```python
from build123d import *

# Parameters (mm, degrees)
F0_R     = 65
F0_R_2   = 5.5
F0_R_3   = 12
F1_DEPTH = 52
F0_R_4   = 81.25
F0_R_5   = 4
F2_DEPTH = 13
F3_DEPTH = 5.2


with BuildPart() as f1:
    # F0 (on Right) → F1 (new body)
    with BuildSketch(Plane.YZ):
        Circle(F0_R)
        with Locations((-28.145826, -16.25)):
            Circle(F0_R_2, mode=Mode.SUBTRACT)
        with Locations((0, -32.5)):
            Circle(F0_R_2, mode=Mode.SUBTRACT)
        with Locations((28.145826, -16.25)):
            Circle(F0_R_2, mode=Mode.SUBTRACT)
        with Locations((-28.145826, 16.25)):
            Circle(F0_R_2, mode=Mode.SUBTRACT)
        Circle(F0_R_3, mode=Mode.SUBTRACT)
        with Locations((28.145826, 16.25)):
            Circle(F0_R_2, mode=Mode.SUBTRACT)
        with Locations((0, 32.5)):
            Circle(F0_R_2, mode=Mode.SUBTRACT)
    extrude(amount=F1_DEPTH)

    # F0 (on Right) → F2 (join)
    with BuildSketch(Plane.YZ):
        Circle(F0_R_4)
        with Locations((-47.013486, -56.028491)):
            Circle(F0_R_5, mode=Mode.SUBTRACT)
        with Locations((-25.015353, -68.729118)):
            Circle(F0_R_5, mode=Mode.SUBTRACT)
        with Locations((-63.341098, -36.57)):
            Circle(F0_R_5, mode=Mode.SUBTRACT)
        with Locations((-72.028839, -12.700628)):
            Circle(F0_R_5, mode=Mode.SUBTRACT)
        with Locations((0, -73.14)):
            Circle(F0_R_5, mode=Mode.SUBTRACT)
        with Locations((25.015353, -68.729118)):
            Circle(F0_R_5, mode=Mode.SUBTRACT)
        with Locations((47.013486, -56.028491)):
            Circle(F0_R_5, mode=Mode.SUBTRACT)
        with Locations((63.341098, -36.57)):
            Circle(F0_R_5, mode=Mode.SUBTRACT)
        with Locations((72.028839, -12.700628)):
            Circle(F0_R_5, mode=Mode.SUBTRACT)
        with Locations((-72.028839, 12.700628)):
            Circle(F0_R_5, mode=Mode.SUBTRACT)
        with Locations((-63.341098, 36.57)):
            Circle(F0_R_5, mode=Mode.SUBTRACT)
        with Locations((-47.013486, 56.028491)):
            Circle(F0_R_5, mode=Mode.SUBTRACT)
        with Locations((-25.015353, 68.729118)):
            Circle(F0_R_5, mode=Mode.SUBTRACT)
        Circle(F0_R, mode=Mode.SUBTRACT)
        with Locations((72.028839, 12.700628)):
            Circle(F0_R_5, mode=Mode.SUBTRACT)
        with Locations((63.341098, 36.57)):
            Circle(F0_R_5, mode=Mode.SUBTRACT)
        with Locations((0, 73.14)):
            Circle(F0_R_5, mode=Mode.SUBTRACT)
        with Locations((25.015353, 68.729118)):
            Circle(F0_R_5, mode=Mode.SUBTRACT)
        with Locations((47.013486, 56.028491)):
            Circle(F0_R_5, mode=Mode.SUBTRACT)
    extrude(amount=F2_DEPTH)

    # F0 (on Right) → F3 (join)
    with BuildSketch(Plane.YZ):
        Circle(F0_R)
        with Locations((-28.145826, -16.25)):
            Circle(F0_R_2, mode=Mode.SUBTRACT)
        with Locations((0, -32.5)):
            Circle(F0_R_2, mode=Mode.SUBTRACT)
        with Locations((28.145826, -16.25)):
            Circle(F0_R_2, mode=Mode.SUBTRACT)
        with Locations((-28.145826, 16.25)):
            Circle(F0_R_2, mode=Mode.SUBTRACT)
        Circle(F0_R_3, mode=Mode.SUBTRACT)
        with Locations((28.145826, 16.25)):
            Circle(F0_R_2, mode=Mode.SUBTRACT)
        with Locations((0, 32.5)):
            Circle(F0_R_2, mode=Mode.SUBTRACT)
    extrude(amount=-F3_DEPTH)


solid = f1.part
```
The listing builds one solid part. Answer for the finished solid, in the listing's coordinates (mm). A direction names the side the tool comes from. Coordinates: 2 decimals unless noted, no trailing zeros. Loops run counter-clockwise (first coordinate to the right, second up) from the corner with the lowest first, then second, coordinate; pieces in that order, holes last. Notation, with made-up numbers: (23.25, -26.75) -> (48.25, -26.75) arc R15 ccw to (48.25, -20.75) -> close; hole circle Ø5 at (68.25, -36.75). An arc over 180 degrees is marked (long way). Return JSON: item names as keys, results as strings. Group by question number.
(1) Find the intervals of material crossed by probe 1 along Z at (x, y) = (11, -0.5); probe 2 along Y at (x, z) = (9, -55); probe 3 along Z at (x, y) = (39, 5), in increasing order. Write a range as from..to.
(2) A cutting plane is placed at C-C on y = -57. Write down the section's boundary in (x, z), and give its area (3 significant figures).
(3) A cutting plane is placed at B-B on z = 30.5. Write down the section's boundary in (x, y), and give its area (3 significant figures).
(4) Determine the mould class of faces 1 (the cylindrical face through (6.409, -25.882, 64.824)), 2 (the cylindrical face through (32.23, 62, 19.52)), 3 (the flat face through (13, -6, -66)) for opening direction Z: released by +Z, released by -Z, zero draft, split by the parting line, or undercut.
(5) Given pin 1 Ø1 at (y, z) = (-54.5, 43) entering from -X; pin 2 Ø3 at (x, y) = (13, 19.5) entering from -Z; pin 3 Ø4 at (x, y) = (21, 45.5) entering from +Z, each flat-ended and moving along its own axis, determine where each tip first touches the part or whether it passes through.
(6) Which of the six approach directions +Z, -Z, +X, -X, +Y, -Y give full straight-line access (tool end or side, diameter ignored) to faces 4 (the flat face through (0, -6, -66)), 5 (the cylindrical face through (6.4, 77.5, 24.4))?
(7) A cutting plane is placed at A-A on x = 32.5. Write down the section's boundary in (y, z), and give its area (3 significant figures).
(8) A cutting plane is placed at D-D on y = 16. Write down the section's boundary in (x, z).
The answers:
{
 "1": {"probe 1": "z = -81.25..-77.11, -69.17..-37.98, -27.02..-11.99, 11.99..27.02, 37.98..69.17, 77.11..81.25", "probe 2": "y = -59.8..-50.88, -43.15..43.15, 50.88..59.8", "probe 3": "z = -64.81..-34.79, -30.21..-10.91, 10.91..30.21, 34.79..64.81"},
 "2": {"outline": "(-5.2, -31.24) -> (0, -31.24) -> (0, -57.9) -> (13, -57.9) -> (13, -31.24) -> (52, -31.24) -> (52, 31.24) -> (13, 31.24) -> (13, 57.9) -> (0, 57.9) -> (0, 31.24) -> (-5.2, 31.24) -> close", "area": "4,270 mm^2"},
 "3": {"outline": "(-5.2, -57.4) -> (0, -57.4) -> (0, -75.31) -> (13, -75.31) -> (13, -57.4) -> (52, -57.4) -> (52, -5.12) -> (-5.2, -5.12) -> close; (-5.2, 5.12) -> (52, 5.12) -> (52, 57.4) -> (13, 57.4) -> (13, 75.31) -> (0, 75.31) -> (0, 57.4) -> (-5.2, 57.4) -> close", "area": "6,450 mm^2"},
 "4": {"face 1": "undercut", "face 2": "split by the parting line", "face 3": "zero draft"},
 "5": {"pin 1": "stops at x = 0", "pin 2": "stops at z = -79.23", "pin 3": "stops at z = 48.3"},
 "6": {"face 4": "-X", "face 5": "+X, -X"},
 "7": {"outline": "circle Ø130 at (0, 0); hole circle Ø11 at (-28.15, -16.25); hole circle Ø11 at (-28.15, 16.25); hole circle Ø24 at (0, 0); hole circle Ø11 at (0, -32.5); hole circle Ø11 at (0, 32.5); hole circle Ø11 at (28.15, -16.25); hole circle Ø11 at (28.15, 16.25)", "area": "12,300 mm^2"},
 "8": {"outline": "(-5.2, -63) -> (0, -63) -> (0, -79.66) -> (13, -79.66) -> (13, -63) -> (52, -63) -> (52, 63) -> (13, 63) -> (13, 79.66) -> (0, 79.66) -> (0, 63) -> (-5.2, 63) -> close"}
}
